Build history of the part. All positions in model axes, mm. Give positions to 0.01 mm unless a question says otherwise; leave off trailing zeros. Order: outer loops, then holes, each group sorted by start corner. A loop starts at its lowest first (then second) coordinate and runs counter-clockwise, first axis right, second up. Notation, with made-up numbers: M 40,-35 L 75,-35 A26 cw 75,-16 Z; hole C 49,78.25 d8. An arc over 180 degrees is marked long. Answer as CSV lines item,"result".
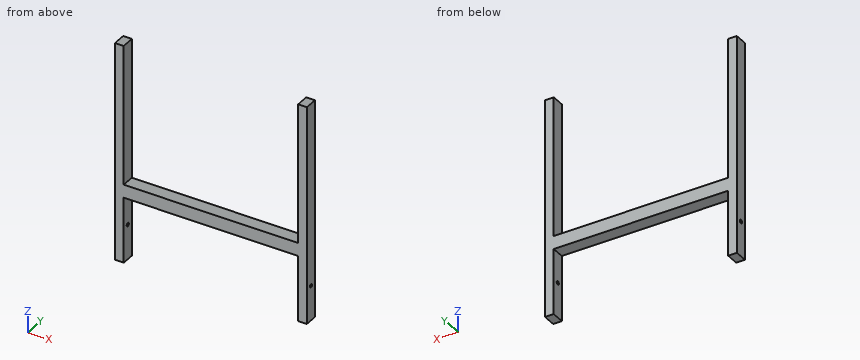
from build123d import *

# Parameters (mm, degrees)
F0_W     = 400
F0_H     = 30
F1_DEPTH = 30
F2_R     = 4
F3_DEPTH = 440.001


with BuildPart() as f1:
    # F0 (on Front) → F1 (new body)
    with BuildSketch(Plane.XZ):
        Polygon((-250, 151.06228), (-270, 151.06228), (-270, -348.93772), (-250, -348.93772), (-250, -198.93772), (-250, -168.93772), align=None)
        with Locations((-50, -183.93772)):
            Rectangle(F0_W, F0_H)
        Polygon((150, 151.06228), (150, -168.93772), (150, -198.93772), (150, -348.93772), (170, -348.93772), (170, 151.06228), align=None)
    extrude(amount=F1_DEPTH)

    # F2 (on face) → F3 (cut, through all)
    with BuildSketch(Plane.YZ.offset(170)):
        with Locations((-15, -268.93772)):
            Circle(F2_R)
    extrude(amount=-F3_DEPTH, mode=Mode.SUBTRACT)


solid = f1.part
Item 1: Band-saw the part on B-B (y = -25.25). Give the cut face in (x, z).
Geometry says:
outline,"M -270,-348.94 L -250,-348.94 L -250,-198.94 L 150,-198.94 L 150,-348.94 L 170,-348.94 L 170,151.06 L 150,151.06 L 150,-168.94 L -250,-168.94 L -250,151.06 L -270,151.06 Z"
Item 2: Drop flat-ended pins along their axis: pin 1 (6 mm diameter, centred on x = 45.5, y = -13.5, fed in from -Z); pin 2 (12 mm diameter, centred on x = -198.5, y = -25, fed in from +Z). Give the stop position or say it passes through.
Geometry says:
pin 1,"stops at z = -198.94"
pin 2,"stops at z = -168.94"
Item 3: Probe line 1 along X through (y, z) = (-2.5, -119.5); line 2 along Z through (x, y) = (-263.5, -15); line 3 along Z through (x, y) = (2, -21.25). List the from-to ranges inside material, lowest first. Write a range as from..to.
Geometry says:
line 1,"x = -270..-250, 150..170"
line 2,"z = -348.94..-272.94, -264.94..151.06"
line 3,"z = -198.94..-168.94"
Item 4: Band-saw the part on A-A (z = -15). Give the cut face in (x, y), and give its area (3 significant figures).
Geometry says:
outline,"M -270,-30 L -250,-30 L -250,0 L -270,0 Z; M 150,-30 L 170,-30 L 170,0 L 150,0 Z"
area,"1,200 mm2"
Item 5: Band-saw the part on C-C (x = 61.5). Give the cut face in (y, z), and give its area (3 significant figures).
Geometry says:
outline,"M -30,-198.94 L 0,-198.94 L 0,-168.94 L -30,-168.94 Z"
area,"900 mm2"
